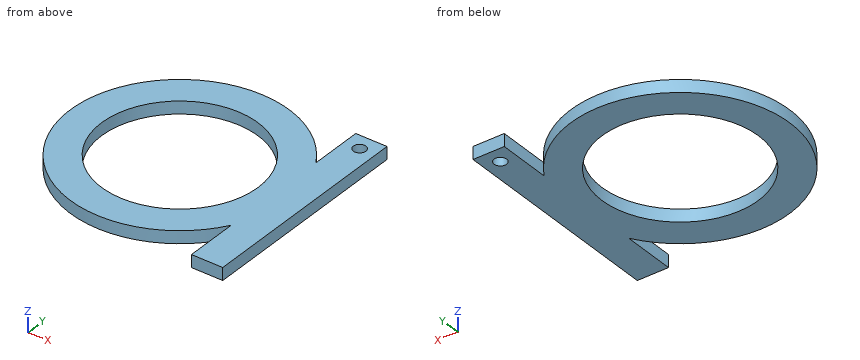
from build123d import *

# Parameters (mm, degrees)
F0_R     = 12.5
F1_DEPTH = 2
F2_R     = 1
F3_DEPTH = 2


with BuildPart() as f1:
    # F0 (on Top) → F1 (new body)
    with BuildSketch(Plane.XY):
        with BuildLine():
            Line((15, -9.0138781887), (15, 9.0138781887))
            ThreePointArc((15, 9.0138781887), (-17.5, 0), (15, -9.0138781887))
        make_face()
        Circle(F0_R, mode=Mode.SUBTRACT)
        with BuildLine():
            ThreePointArc((15, -9.0138781887), (16.863421954, -4.6770717335), (17.5, 0))
            ThreePointArc((17.5, 0), (16.863421954, 4.6770717335), (15, 9.0138781887))
            Line((15, 9.0138781887), (15, -9.0138781887))
        make_face()
        with BuildLine():
            ThreePointArc((15, 9.0138781887), (16.863421954, 4.6770717335), (17.5, 0))
            ThreePointArc((17.5, 0), (16.863421954, -4.6770717335), (15, -9.0138781887))
            Line((15, -9.0138781887), (15, -17.5))
            Line((15, -17.5), (20, -17.5))
            Line((20, -17.5), (20, 17.5))
            Line((20, 17.5), (15, 17.5))
            Line((15, 17.5), (15, 9.0138781887))
        make_face()
    extrude(amount=F1_DEPTH)

    # F2 (on face) → F3 (cut)
    with BuildSketch(Plane.XY.offset(2)):
        with Locations((17.5, 15)):
            Circle(F2_R)
    extrude(amount=-F3_DEPTH, mode=Mode.SUBTRACT)


solid = f1.part
Can you work these out from the model? Positions are in its coordinate system, mm. Give positions to 0.01 mm unless a question says otherwise; leave off trailing zeros. Write each loop counter-clockwise with the first axis right and the second up, starting at its lowest first coordinate (ties: lowest second). Pieces come first, ordered by that corner, then holes. Notation, with made-up numbers: (-17, 10) -> (-4, 10) arc R25 ccw to (-4, 33) -> close; hole circle Ø6 at (-32, 5). An arc over 180 degrees is marked (long way). Answer as a JSON object with one key per item and string values. Group by question number.
Item 1: Suppose I cut it at C-C (y = 15). Please give me the cut outline in (x, z).
Item 2: Please list where these lines run through material, in increasing order: line 1 (X direction, y = 11.5, z = 0.5); line 2 (Y direction, x = 17.5, z = 0.95); line 3 (Y direction, x = 0, z = 1.45). Write a range as [from, to].
Item 3: Suppose I cut it at A-A (y = 0). Please give me the cut outline in (x, z).
Item 4: Suppose I cut it at D-D (z = 0.7). Please give me the cut outline in (x, y), plus the area to 3 significant figures.
Item 5: Suppose I cut it at B-B (x = -7). Please give me the cut outline in (y, z), plus the area to 3 significant figures.
Item 6: I'm going to push a flat-ended pin straight in: P1, Ø1, axis at y = 4, z = 0.5, coming from the -X side. Where does the tip first touch, or does it pass through?
Findings:
{
 "1": {"outline": "(-9.01, 0) -> (9.01, 0) -> (9.01, 2) -> (-9.01, 2) -> close; (15, 0) -> (16.5, 0) -> (16.5, 2) -> (15, 2) -> close; (18.5, 0) -> (20, 0) -> (20, 2) -> (18.5, 2) -> close"},
 "2": {"line 1": "x = [-13.19, -4.9], [4.9, 13.19], [15, 20]", "line 2": "y = [-17.5, 14], [16, 17.5]", "line 3": "y = [-17.5, -12.5], [12.5, 17.5]"},
 "3": {"outline": "(-17.5, 0) -> (-12.5, 0) -> (-12.5, 2) -> (-17.5, 2) -> close; (12.5, 0) -> (20, 0) -> (20, 2) -> (12.5, 2) -> close"},
 "4": {"outline": "(15, -17.5) -> (20, -17.5) -> (20, 17.5) -> (15, 17.5) -> (15, 9.01) arc R17.5 ccw (long way) to (15, -9.01) -> close; hole circle Ø25 at (0, 0); hole circle Ø2 at (17.5, 15)", "area": "613 mm²"},
 "5": {"outline": "(-16.04, 0) -> (-10.36, 0) -> (-10.36, 2) -> (-16.04, 2) -> close; (10.36, 0) -> (16.04, 0) -> (16.04, 2) -> (10.36, 2) -> close", "area": "22.7 mm²"},
 "6": {"P1": "stops at x = -17.15"}
}
